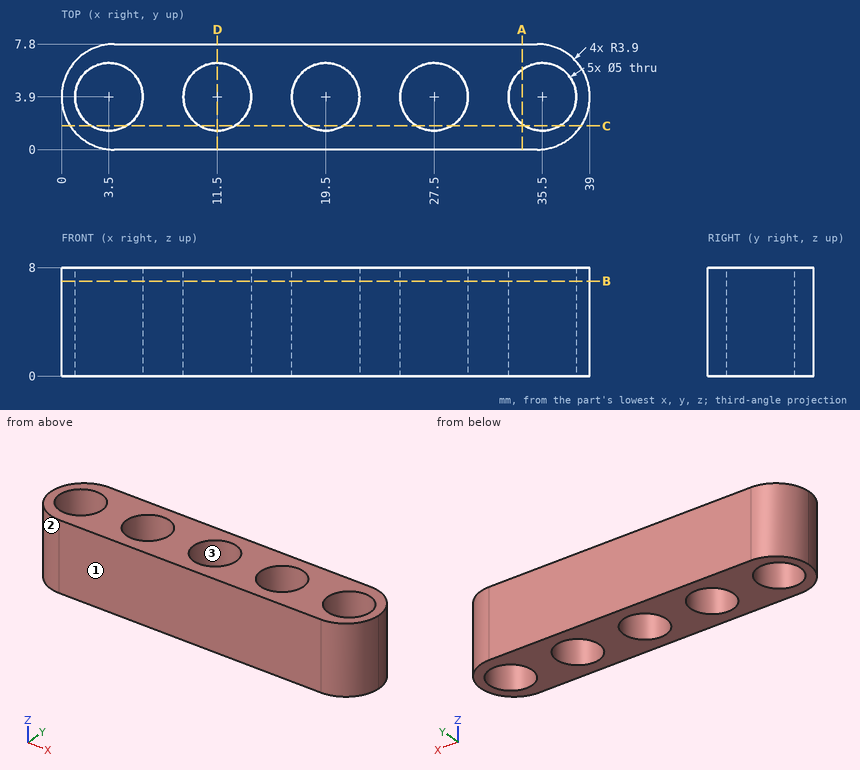
Job drawing, mm, ordinate dimensions from the low corner. One solid piece. Round coordinates to 2 decimals unless told otherwise and drop trailing zeros. Write each loop counter-clockwise with the first axis right and the second up, starting at its lowest first coordinate (ties: lowest second). Pieces come first, ordered by that corner, then holes. Notation, with made-up numbers: (23.5, 49.5) -> (32.5, 49.5) arc R20 ccw to (32.5, 53.5) -> close; hole circle Ø3 at (51.5, 16.25). An arc over 180 degrees is marked (long way). Answer as a JSON object with one key per item and string values.
(1) Pin check, flat tip, straight feed: P1, Ø4.5, axis at x = 35.5, y = 3.9, coming from the +Z side. Stop position of the tip, or through.
Reported:
{"P1": "passes through"}
(2) Probe probe 1 along X at (y, z) = (4, 6.75); probe 2 along X at (y, z) = (2.5, 5.5); probe 3 along X at (y, z) = (6.5, 5.75) (1 decimal). List the from-to ranges inside material, lowest first. Write a range as [from, to].
Reported:
{"probe 1": "x = [0, 1], [6, 9], [14, 17], [22, 25], [30, 33], [38, 39]", "probe 2": "x = [0.26, 1.43], [5.57, 9.43], [13.57, 17.43], [21.57, 25.43], [29.57, 33.43], [37.57, 38.74]", "probe 3": "x = [1, 38]"}
(3) Band-saw the part on C-C, the plane y = 1.75. List the corners of the cut face in (x, z) (1 decimal).
Reported:
{"outline": "(0.6, 0) -> (2.2, 0) -> (2.2, 8) -> (0.6, 8) -> close; (4.8, 0) -> (10.2, 0) -> (10.2, 8) -> (4.8, 8) -> close; (12.8, 0) -> (18.2, 0) -> (18.2, 8) -> (12.8, 8) -> close; (20.8, 0) -> (26.2, 0) -> (26.2, 8) -> (20.8, 8) -> close; (28.8, 0) -> (34.2, 0) -> (34.2, 8) -> (28.8, 8) -> close; (36.8, 0) -> (38.4, 0) -> (38.4, 8) -> (36.8, 8) -> close"}
(4) Two-plate mould, pull along X, no slides. Class the marked faces 1, 2 and 3: +X half, -X half, draft (parallel to the pull), parting line (faces both ways), or undercut.
Reported:
{"face 1": "draft", "face 2": "-X half", "face 3": "undercut"}
(5) Band-saw the part on D-D, the plane x = 11.5. List the corners of the cut face in (y, z), then the cut area to 3 significant figures.
Reported:
{"outline": "(0, 0) -> (1.4, 0) -> (1.4, 8) -> (0, 8) -> close; (6.4, 0) -> (7.8, 0) -> (7.8, 8) -> (6.4, 8) -> close", "area": "22.4 mm^2"}
(6) Band-saw the part on A-A, the plane x = 34. List the corners of the cut face in (y, z), then the cut area to 3 significant figures.
Reported:
{"outline": "(0, 0) -> (1.9, 0) -> (1.9, 8) -> (0, 8) -> close; (5.9, 0) -> (7.8, 0) -> (7.8, 8) -> (5.9, 8) -> close", "area": "30.4 mm^2"}
(7) Band-saw the part on B-B, the plane z = 7. Count the separate pieces of the cut face and the enclosed holes in it, then the cut area to 3 significant figures.
Reported:
{"separate pieces": "1", "enclosed holes": "5", "area": "193 mm^2"}
